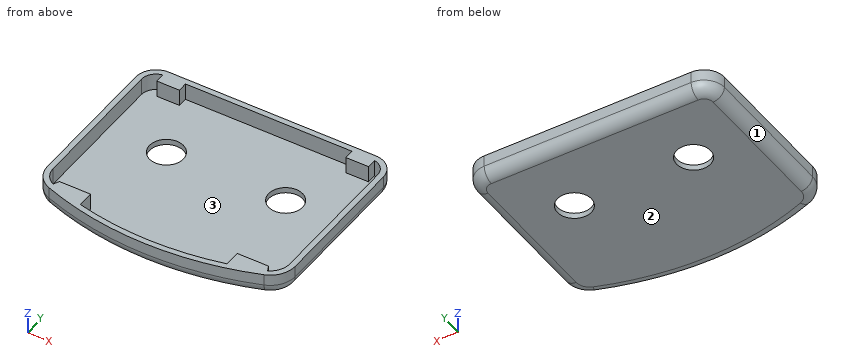
from build123d import *

# Parameters (mm, degrees)
F1_DEPTH = 12.7
F2_T     = -3.175
F3_R     = 6.35
F5_W     = 12.7
F5_H     = 6.35
F6_DEPTH = 9.398
F7_R     = 9.525
F8_DEPTH = 25.4


# Not quite as in the source:
# - a feature names something its author has since deleted; it is built from what else it names


with BuildPart() as f1:
    # F0 (on Top) → F1 (new body)
    with BuildSketch(Plane.XY):
        with BuildLine():
            Line((58.0965084505, 62.5356453779), (-58.0965084505, 62.5356453779))
            ThreePointArc((-58.0965084505, 62.5356453779), (-66.1787389595, 59.1878758868), (-69.5265084505, 51.1056453779))
            Line((-69.5265084505, 51.1056453779), (-69.5265084505, -27.1992570698))
            ThreePointArc((-69.5265084505, -27.1992570698), (-67.0115325937, -35.1957139026), (-60.3721316603, -40.3130159932))
            ThreePointArc((-60.3721316603, -40.3130159932), (0, -51.0474727306), (60.3721316603, -40.3130159932))
            ThreePointArc((60.3721316603, -40.3130159932), (67.0115325937, -35.1957139026), (69.5265084505, -27.1992570698))
            Line((69.5265084505, -27.1992570698), (69.5265084505, 51.1056453779))
            ThreePointArc((69.5265084505, 51.1056453779), (66.1787389595, 59.1878758868), (58.0965084505, 62.5356453779))
        make_face()
    extrude(amount=F1_DEPTH)

    # F2
    f2_openings = [f1.faces().sort_by_distance(p)[0] for p in [
        (0, 7.919531, 12.7),
    ]]
    offset(amount=F2_T, openings=f2_openings)

    # F3
    f3_edges = [f1.edges().sort_by_distance(p)[0] for p in [
        (69.526508, 11.953194, 0),
        (66.178739, 59.187876, 0),
        (0, 62.535645, 0),
        (-66.178739, 59.187876, 0),
        (-69.526508, 11.953194, 0),
        (-67.011533, -35.195714, 0),
        (0, -51.047473, 0),
        (67.011533, -35.195714, 0),
    ]]
    fillet(f3_edges, radius=F3_R)

    # F5 (on offset) → F6 (join)
    with BuildSketch(Plane.XY.offset(12.7)):
        with Locations((-53.0805146158, 57.0815077901)):
            Rectangle(F5_W, F5_H)
        with Locations((53.0805146158, 57.0815077901)):
            Rectangle(F5_W, F5_H)
        Polygon((-41.1868803203, -33.773638308), (-58.6946308613, -33.773638308), (-60.6418885291, -37.9110425711), (-53.9016760886, -40.266495198), (-41.1868803203, -43.3214269578), align=None)
        Polygon((60.6418885291, -37.9110425711), (58.6946308613, -33.773638308), (41.1868803203, -33.773638308), (41.1868803203, -43.3214269578), (53.9016760886, -40.266495198), align=None)
    extrude(amount=-F6_DEPTH)

    # F7 (on face) → F8 (cut)
    with BuildSketch(Plane.XY.offset(3.175)):
        with Locations((-33.4585084505, 21.3863216341)):
            Circle(F7_R)
        with Locations((33.4585084505, 21.3863216341)):
            Circle(F7_R)
    extrude(amount=-F8_DEPTH, mode=Mode.SUBTRACT)


solid = f1.part
Here's how the part is built. I have some questions about the finished solid (model axes, mm). Face numbers are marked on the shaded views. Round coordinates to 2 decimals unless told otherwise and drop trailing zeros. Order: outer loops, then holes, each group sorted by start corner. A loop starts at its lowest first (then second) coordinate and runs counter-clockwise, first axis right, second up. Notation, with made-up numbers: M 1.5,60 L 58.5,60 A24 ccw 58.5,97 Z; hole C 79.25,-8.5 d4. An arc over 180 degrees is marked long. Return JSON: item names as keys, results as strings. Group by question number.
1. I'm going to push flat-ended pins straight in: pin 1 Ø15 at (x, y) = (33.46, 21.39) entering from +Z; pin 2 Ø4.5 at (y, z) = (-40.5, 6.5) entering from +X; pin 3 Ø10 at (x, y) = (49.5, -37) entering from -Z; pin 4 Ø3 at (x, z) = (-54, 9) entering from -Y. Where does each tip first touch, or does it pass through?
2. If we section it at A-A on z = 9.75: List the corners of the cut face in (x, y) for me (1 decimal), then the cut area to 3 significant figures.
3. If we mould it in two halves opening along X, with no side actions, what happens to the marked faces 1, 2 and 3? For each: pulls with the +X half, pulls with the -X half, needs draft (parallel to the pull), parting line crosses it, or undercut.
4. Please list where these lines run through material, in increasing order: probe 1 along X at (y, z) = (9, 6.25); probe 2 along X at (y, z) = (56, 9); probe 3 along Y at (x, z) = (-3, 11).
Reply:
{
 "1": {"pin 1": "through", "pin 2": "x = 64.1", "pin 3": "z = 0", "pin 4": "y = -42.99"},
 "2": {"outline": "M -69.5,-27.2 A14 ccw -60.4,-40.3 A175.1 ccw 60.4,-40.3 A14 ccw 69.5,-27.2 L 69.5,51.1 A11.4 ccw 58.1,62.5 L -58.1,62.5 A11.4 ccw -69.5,51.1 Z; hole M -66.4,-27.2 A10.8 ccw -60.2,-36.9 L -58.7,-33.8 L -41.2,-33.8 L -41.2,-42.9 A172 ccw 41.2,-42.9 L 41.2,-33.8 L 58.7,-33.8 L 60.2,-36.9 A10.8 ccw 66.4,-27.2 L 66.4,51.1 A8.3 ccw 59.4,59.3 L 59.4,53.9 L 46.7,53.9 L 46.7,59.4 L -46.7,59.4 L -46.7,53.9 L -59.4,53.9 L -59.4,59.3 A8.3 ccw -66.4,51.1 Z", "area": "1,820 mm^2"},
 "3": {"face 1": "pulls with the -X half", "face 2": "needs draft", "face 3": "undercut"},
 "4": {"probe 1": "-69.53 to -66.35, 66.35 to 69.53", "probe 2": "-68.43 to -64.74, -59.43 to -46.73, 46.73 to 59.43, 64.74 to 68.43", "probe 3": "-51.02 to -47.85, 59.36 to 62.54"}
}
